Geometry check sheet. Reference: drawing and pictorial views, mm from the part's lowest x, y, z. Give positions to 0.01 mm unless a question says otherwise; leave off trailing zeros. Order: outer loops, then holes, each group sorted by start corner. A loop starts at its lowest first (then second) coordinate and runs counter-clockwise, first axis right, second up.
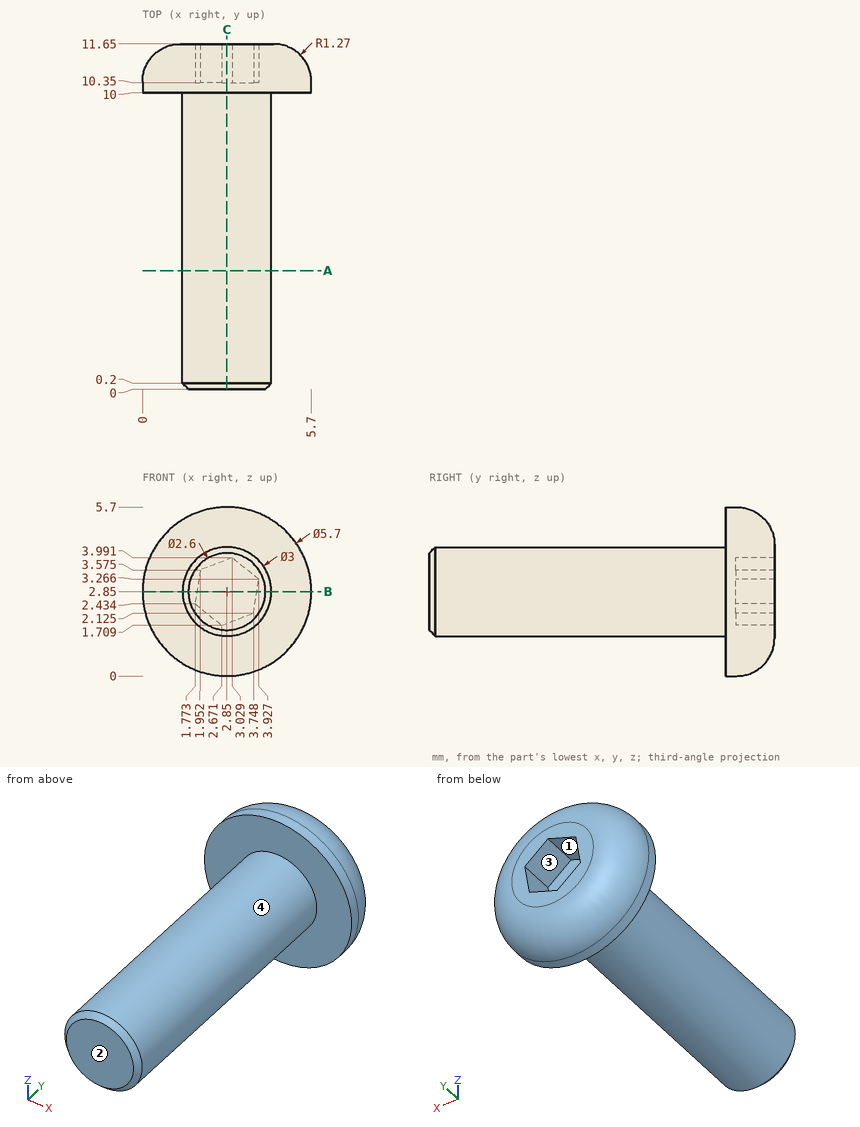
(1) Cross-section at C-C on x = 2.85. Enter the section's corners in (y, z).
Response values:
outline: (0, 1.55) - (0.2, 1.35) - (10, 1.35) - (10, 0) - (10.38, 0) arc R1.27 ccw to (11.65, 1.27) - (11.65, 1.78) - (10.35, 1.78) - (10.35, 3.92) - (11.65, 3.92) - (11.65, 4.43) arc R1.27 ccw to (10.38, 5.7) - (10, 5.7) - (10, 4.35) - (0.2, 4.35) - (0, 4.15) - close
(2) Material ranges on L1, parallel to Y at x = 4.35, z = 3.55; L2, parallel to Z at x = 1.65, y = 1; L3, parallel to Y at x = 3.4, z = 2.6, recorded low to high.
Response values:
L1: y = 10 to 11.65
L2: z = 1.95 to 3.75
L3: y = 0 to 10.35
(3) Cross-section at A-A on y = 4. Enter the section's corners in (x, z).
Response values:
outline: circle Ø3 at (2.85, 2.85)
(4) Release check for a two-part mould opening along X. For the marked faces 1, 2, 3 and 4 record: released by +X, released by -X, zero draft, split by the parting line, or undercut.
Response values:
face 1: undercut
face 2: zero draft
face 3: undercut
face 4: split by the parting line
(5) Gauge pin test, flat end, axial feed: pin 1 Ø1 at (x, y) = (2.5, 2.5) entering from +Z. Record the tip position at first contact, or that the pin passes through.
Response values:
pin 1: stops at z = 4.35
(6) Cross-section at B-B on z = 2.85. Enter the section's corners in (x, y).
Response values:
outline: (0, 10) - (1.35, 10) - (1.35, 0.2) - (1.55, 0) - (4.15, 0) - (4.35, 0.2) - (4.35, 10) - (5.7, 10) - (5.7, 10.38) arc R1.27 ccw to (4.43, 11.65) - (3.86, 11.65) - (3.86, 10.35) - (1.84, 10.35) - (1.84, 11.65) - (1.27, 11.65) arc R1.27 ccw to (0, 10.38) - close
